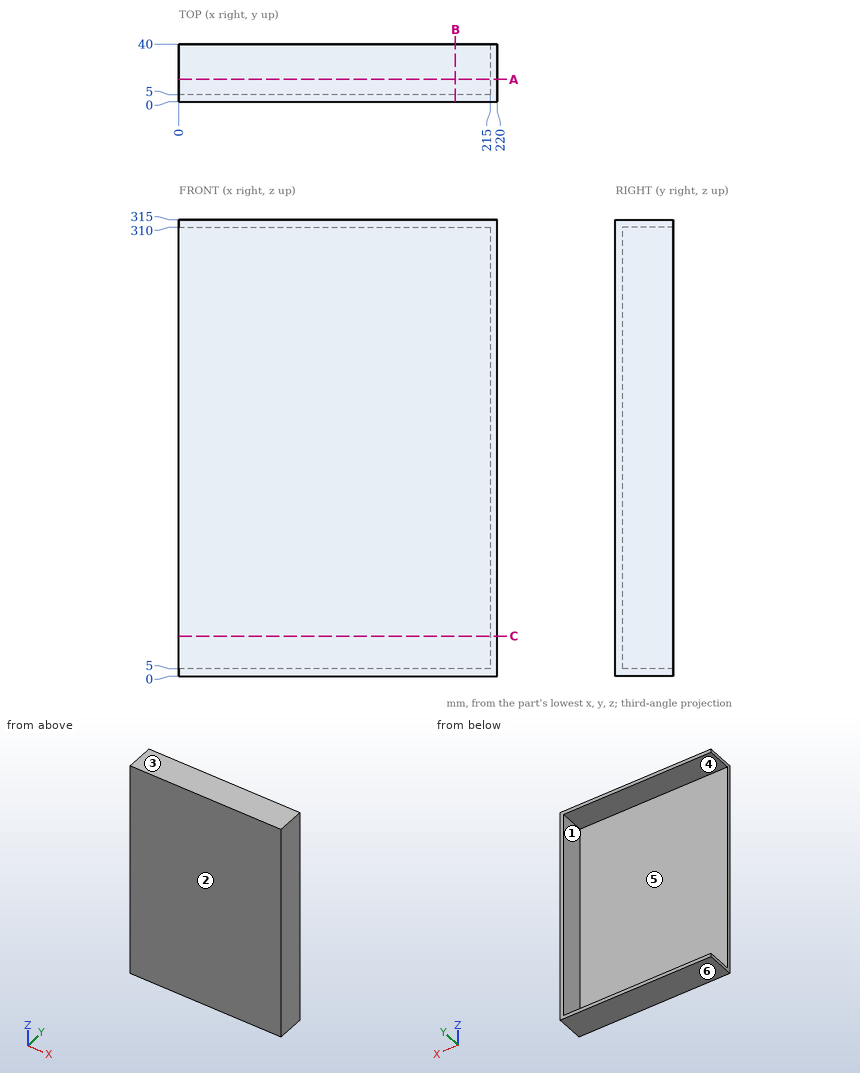
Study the drawing (mm; zero at the part's minimum x, y, z) and answer. A direction names the side the tool comes from. Round coordinates to 2 decimals unless told otherwise and drop trailing zeros. Loops run counter-clockwise (first coordinate to the right, second up) from the corner with the lowest first, then second, coordinate; pieces in that order, holes last.
Q1. Find the intervals of material crossed by line 1 (Z direction, x = 112, y = 37.5); line 2 (Y direction, x = 38, z = 117); line 3 (X direction, y = 20, z = 115), in increasing order.
Q2. For a pull along Z with two mould halves and no side action, classify the marked faces 1, 2, 3 and 4 as released by +Z, released by -Z, zero draft, split by the parting line, or undercut.
Q3. Section A-A, the plane y = 15.5 is taken. Determine the outline of the cut face in (x, z), then the cut area to 4 significant figures.
Q4. Section C-C, the plane z = 27.5 is taken. Determine the outline of the cut face in (x, y).
Q5. Which of the six approach directions +Z, -Z, +X, -X, +Y, -Y give full straight-line access (tool end or side, diameter ignored) to the marked faces 5 and 6?
Q6. Section B-B, the plane x = 191 is taken. Determine the outline of the cut face in (y, z).
Q7. Given pin 1 Ø8 at (x, y) = (181, 28.5) entering from -Z; pin 2 Ø3 at (y, z) = (23, 94) entering from -X; pin 3 Ø12 at (x, z) = (183, 173.5) entering from +Y, each flat-ended and moving along its own axis, determine where each tip first touches the part or whether it passes through.
Completed:
1. line 1: z = 0 to 5, 310 to 315
1. line 2: y = 0 to 5
1. line 3: x = 215 to 220
2. face 1: undercut
2. face 2: zero draft
2. face 3: released by +Z
2. face 4: undercut
3. outline: (0, 0) - (220, 0) - (220, 315) - (0, 315) - (0, 310) - (215, 310) - (215, 5) - (0, 5) - close
3. area: 3,725 mm2
4. outline: (0, 0) - (220, 0) - (220, 40) - (215, 40) - (215, 5) - (0, 5) - close
5. face 5: -X, +Y
5. face 6: -Z, +X, -X, +Y, -Y
6. outline: (0, 0) - (40, 0) - (40, 5) - (5, 5) - (5, 310) - (40, 310) - (40, 315) - (0, 315) - close
7. pin 1: stops at z = 0
7. pin 2: stops at x = 215
7. pin 3: stops at y = 5
